```python
from build123d import *

# Parameters (mm, degrees)
ESBO_O1_W                = 62.4
ESBO_O1_H                = 75
RESSALTO_EXTRUS_O1_DEPTH = 2
ESBO_O2_W                = 75
ESBO_O2_H                = 40
RESSALTO_EXTRUS_O2_DEPTH = 2
ESBO_O3_R                = 2.5
CORTE_EXTRUS_O1_DEPTH    = 67.4
ESBO_O4_R                = 20
CORTE_EXTRUS_O2_DEPTH    = 5
ESBO_O5_R                = 2.75
CORTE_EXTRUS_O3_DEPTH    = 3
ESBO_O11_W               = 75
ESBO_O11_H               = 40
RESSALTO_EXTRUS_O3_DEPTH = 67.85
ESBO_O12_W               = 75
ESBO_O12_H               = 38
CORTE_EXTRUS_O4_DEPTH    = 67.85
ESBO_O13_R               = 2.5
CORTE_EXTRUS_O5_DEPTH    = 64.1
ESBO_O14_R               = 7.5
CORTE_EXTRUS_O6_DEPTH    = 10
CORTE_EXTRUS_O7_DEPTH    = 10
ESBO_O17_R               = 4
CORTE_EXTRUS_O8_DEPTH    = 10


with BuildPart() as part:
    # Esboço1 → Ressalto-extrusão1 (new body)
    with BuildSketch(Plane(origin=(0, 0, 0), x_dir=(1, 0, 0), z_dir=(0, 1, 0))):
        Rectangle(ESBO_O1_W, ESBO_O1_H)
    extrude(amount=RESSALTO_EXTRUS_O1_DEPTH)

    # Esboço2 → Ressalto-extrusão2 (add)
    with BuildSketch(Plane(origin=(31.2, 0, 0), x_dir=(0, 0, -1), z_dir=(1, 0, 0))):
        with Locations((0, 20)):
            Rectangle(ESBO_O2_W, ESBO_O2_H)
    ressalto_extrus_o2 = extrude(amount=RESSALTO_EXTRUS_O2_DEPTH)

    # Espelhar1: Ressalto-extrusão2 across plane
    add(ressalto_extrus_o2.mirror(Plane(origin=(0, 0, 0), x_dir=(0, 0, 1), z_dir=(1, 0, 0))))

    # Esboço3 → Corte-extrusão1 (cut, through all)
    with BuildSketch(Plane.ZY.offset(33.2)):
        with Locations((-28.5, 29)):
            Circle(ESBO_O3_R)
        with Locations((28.5, 29)):
            Circle(ESBO_O3_R)
    extrude(amount=-CORTE_EXTRUS_O1_DEPTH, mode=Mode.SUBTRACT)

    # Esboço4 → Corte-extrusão2 (cut)
    with BuildSketch(Plane(origin=(0, 2, 0), x_dir=(1, 0, 0), z_dir=(0, 1, 0))):
        Circle(ESBO_O4_R)
    extrude(amount=-CORTE_EXTRUS_O2_DEPTH, mode=Mode.SUBTRACT)

    # Esboço5 → Corte-extrusão3 (cut, through all)
    with BuildSketch(Plane(origin=(0, 2, 0), x_dir=(1, 0, 0), z_dir=(0, 1, 0))):
        with Locations((23.57, 23.57)):
            Circle(ESBO_O5_R)
        with Locations((23.57, -23.57)):
            Circle(ESBO_O5_R)
        with Locations((-23.57, -23.57)):
            Circle(ESBO_O5_R)
        with Locations((-23.57, 23.57)):
            Circle(ESBO_O5_R)
    extrude(amount=-CORTE_EXTRUS_O3_DEPTH, mode=Mode.SUBTRACT)

    # Esboço11 → Ressalto-extrusão3 (add)
    with BuildSketch(Plane.ZY.offset(33.2)):
        with Locations((0, 20)):
            Rectangle(ESBO_O11_W, ESBO_O11_H)
    extrude(amount=RESSALTO_EXTRUS_O3_DEPTH)

    # Esboço12 → Corte-extrusão4 (cut)
    with BuildSketch(Plane(origin=(-31.2, 0, 0), x_dir=(0, 0, -1), z_dir=(1, 0, 0))):
        with Locations((0, 21)):
            Rectangle(ESBO_O12_W, ESBO_O12_H)
    extrude(amount=-CORTE_EXTRUS_O4_DEPTH, mode=Mode.SUBTRACT)

    # Esboço13 → Corte-extrusão5 (cut)
    with BuildSketch(Plane(origin=(-99.05, 0, 0), x_dir=(0, 0, -1), z_dir=(1, 0, 0))):
        with Locations((28.5, 29)):
            Circle(ESBO_O13_R)
        with Locations((-28.5, 29)):
            Circle(ESBO_O13_R)
    extrude(amount=-CORTE_EXTRUS_O5_DEPTH, mode=Mode.SUBTRACT)

    # Esboço14 → Corte-extrusão6 (cut)
    with BuildSketch(Plane(origin=(0, 2, 0), x_dir=(1, 0, 0), z_dir=(0, 1, 0))):
        with Locations((-54, 0)):
            Circle(ESBO_O14_R)
    extrude(amount=-CORTE_EXTRUS_O6_DEPTH, mode=Mode.SUBTRACT)

    # Esboço16 → Corte-extrusão7 (cut)
    with BuildSketch(Plane(origin=(0, 2, 0), x_dir=(1, 0, 0), z_dir=(0, 1, 0))):
        with BuildLine():
            ThreePointArc((-57.5, 26.5), (-54, 23), (-50.5, 26.5))
            ThreePointArc((-50.5, 26.5), (-54, 30), (-57.5, 26.5))
        make_face()
        with BuildLine():
            ThreePointArc((-50.5, -26.5), (-54, -23), (-57.5, -26.5))
            ThreePointArc((-57.5, -26.5), (-54, -30), (-50.5, -26.5))
        make_face()
    extrude(amount=-CORTE_EXTRUS_O7_DEPTH, mode=Mode.SUBTRACT)

    # Esboço17 → Corte-extrusão8 (cut)
    with BuildSketch(Plane.ZY.offset(-31.2)):
        with Locations((0, 20)):
            Circle(ESBO_O17_R)
    extrude(amount=-CORTE_EXTRUS_O8_DEPTH, mode=Mode.SUBTRACT)


solid = part.part
```
Source: CAD feature listing. Evaluate the final solid. Frame: model axes, mm. A direction names the side the tool comes from. Coordinates: 2 decimals unless noted, no trailing zeros. Loops run counter-clockwise (first coordinate to the right, second up) from the corner with the lowest first, then second, coordinate; pieces in that order, holes last. Notation, with made-up numbers: (10.25, -10.5) -> (27.25, -10.5) arc R36 cw to (27.25, 28.5) -> close; hole circle Ø9 at (76, 17.5). An arc over 180 degrees is marked (long way). One line per item, written item: value. Start each with the question number.
Q1. Section query B-B, the plane z = 16. Return the cut outline in (x, y).
Q2. Set-up query: faces 5 (the face through (32.19, 31.48, -28.83)), 6 (the face through (32.186, 23.966, -0.521)), 7 (the face through (31.2, 25, 1)). Return all of +Z, -Z, +X, -X, +Y, -Y with unobstructed straight access to the full face (end or side cutting, diameter ignored); none if empty.
Q3. Mould query, pull axis Z, two halves, no side actions, for faces 1 (the face through (33.2, 15.8, 0.5)), 2 (the face through (-34, 1, 37.5)), 3 (the face through (32.19, 31.48, 28.17)), 4 (the face through (-100.04, 31.48, 28.83)). Classes: pulls with the +Z half, pulls with the -Z half, needs draft (parallel to the pull), parting line crosses it, or undercut.
Q4. Line query: line 1 along X through (y, z) = (1.6, 0); line 2 along X through (y, z) = (34.5, -29.5); line 3 along X through (y, z) = (1.3, -26.5). Output: solid intervals per line, ascending.
Q5. Contact query for a flat-ended pin moving along its axis: P1, Ø24, axis at x = -54, z = 0, coming from the +Y side. Output: stop coordinate, or through.
Q6. Section query D-D, the plane y = 10. Return the cut outline in (x, z), and give its area (3 significant figures).
Q7. Section query A-A, the plane y = 29. Return the cut outline in (x, z).
Q8. Section query C-C, the plane x = 12. Return the cut outline in (y, z), and give its area (3 significant figures).
Results:
1. outline: (-101.05, 0) -> (-12, 0) -> (-12, 2) -> (-99.05, 2) -> (-99.05, 40) -> (-101.05, 40) -> close; (12, 0) -> (33.2, 0) -> (33.2, 40) -> (31.2, 40) -> (31.2, 2) -> (12, 2) -> close
2. face 5: +X, -X
2. face 6: +X
2. face 7: +Z, -Z, +Y
3. face 1: needs draft
3. face 2: pulls with the +Z half
3. face 3: undercut
3. face 4: undercut
4. line 1: -101.05 to -61.5, -46.5 to -20, 20 to 33.2
4. line 2: -101.05 to -99.05, 31.2 to 33.2
4. line 3: -101.05 to -57.5, -50.5 to 33.2
5. P1: y = 2
6. outline: (-101.05, -37.5) -> (-99.05, -37.5) -> (-99.05, 37.5) -> (-101.05, 37.5) -> close; (31.2, -37.5) -> (33.2, -37.5) -> (33.2, 37.5) -> (31.2, 37.5) -> close
6. area: 300 mm^2
7. outline: (-101.05, -37.5) -> (-99.05, -37.5) -> (-99.05, -31) -> (-101.05, -31) -> close; (-101.05, -26) -> (-99.05, -26) -> (-99.05, 26) -> (-101.05, 26) -> close; (-101.05, 31) -> (-99.05, 31) -> (-99.05, 37.5) -> (-101.05, 37.5) -> close; (31.2, -37.5) -> (33.2, -37.5) -> (33.2, -31) -> (31.2, -31) -> close; (31.2, -26) -> (33.2, -26) -> (33.2, 26) -> (31.2, 26) -> close; (31.2, 31) -> (33.2, 31) -> (33.2, 37.5) -> (31.2, 37.5) -> close
8. outline: (0, -37.5) -> (2, -37.5) -> (2, -16) -> (0, -16) -> close; (0, 16) -> (2, 16) -> (2, 37.5) -> (0, 37.5) -> close
8. area: 86.0 mm^2
